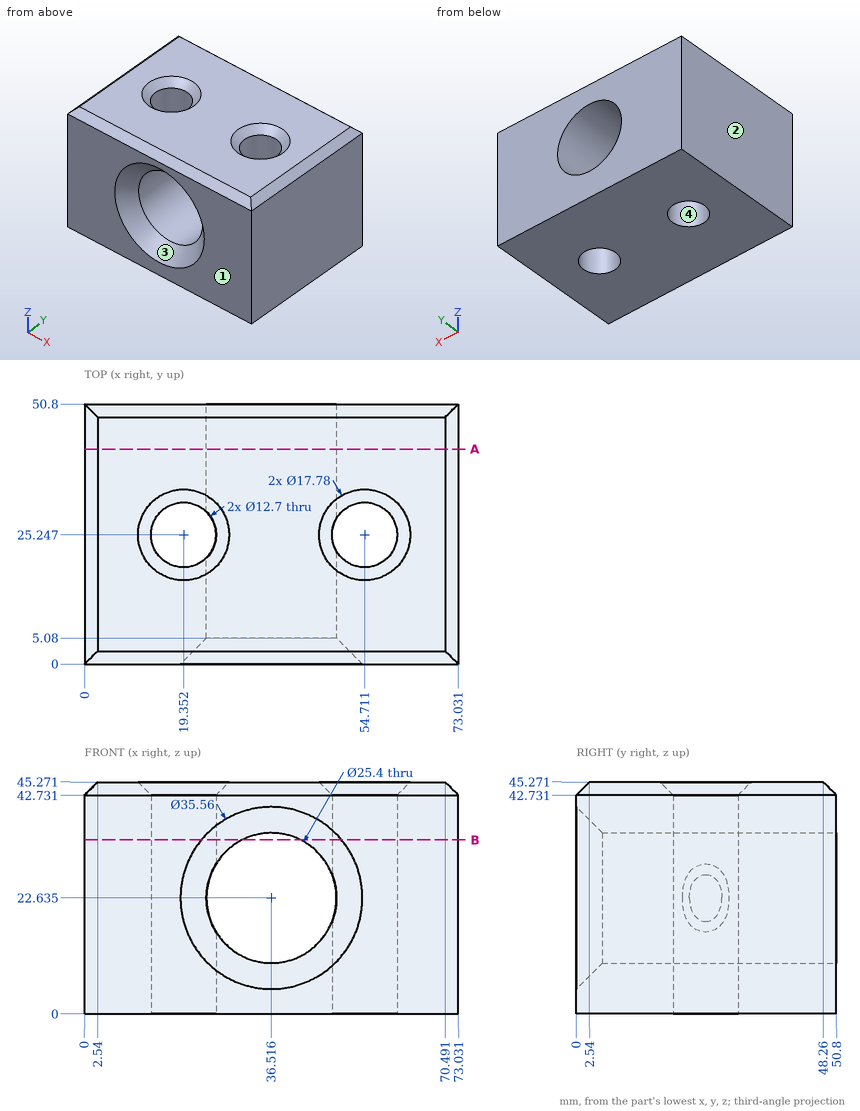
Input: dimensioned drawing with shaded views. Units: mm. Origin: part minimum x, y, z. Round coordinates to 2 decimals unless told otherwise and drop trailing zeros. Loops run counter-clockwise (first coordinate to the right, second up) from the corner with the lowest first, then second, coordinate; pieces in that order, holes last. Notation, with made-up numbers: M 72,3.25 L 81,3.25 A22 ccw 81,9.25 Z; hole C -8,-21.5 d7. An arc over 180 degrees is marked long. Return JSON: item names as keys, results as strings. Group by question number.
1. Mould query, pull axis X, two halves, no side actions, for the marked faces 1, 2, 3 and 4. Classes: released by +X, released by -X, zero draft, split by the parting line, or undercut.
2. Section query B-B on z = 34. State how many separate pieces and enclosed holes the cut face has, and give its area (3 significant figures).
3. Section query A-A on y = 42. Output: boundary loops of the cut face in (x, z) (1 decimal).
4. Material intervals for line 1 along X through (y, z) = (21, 23); line 2 along X through (y, z) = (26.5, 3.5); line 3 along Z through (x, y) = (36, 35.5) (1 decimal), sorted ascending. Write a range as from..to.
5. Pin query (flat end, axial travel): pin 1 (12 mm diameter, centred on x = 57.5, z = 39.5, fed in from -Y). Return the tip coordinate at first contact, or that it passes through.
Checks:
{
 "1": {"face 1": "zero draft", "face 2": "released by -X", "face 3": "undercut", "face 4": "undercut"},
 "2": {"separate pieces": "2", "enclosed holes": "2", "area": "2,840 mm²"},
 "3": {"outline": "M 0,0 L 73,0 L 73,42.7 L 70.5,45.3 L 2.5,45.3 L 0,42.7 Z; hole C 36.5,22.6 d25.4"},
 "4": {"line 1": "x = 0..14.63, 49.21..49.99, 59.43..73.03", "line 2": "x = 0..13.13, 25.58..48.49, 60.94..73.03", "line 3": "z = 0..9.9, 35.3..45.3"},
 "5": {"pin 1": "stops at y = 0"}
}
